The figure shows three views and two pictorial views of one solid part (mm, origin at its lowest corner). Answer the questions. Give positions to 0.01 mm unless a question says otherwise; leave off trailing zeros. Order: outer loops, then holes, each group sorted by start corner. A loop starts at its lowest first (then second) coordinate and runs counter-clockwise, first axis right, second up. Notation, with made-up numbers: M 27,50.5 L 41,50.5 A13 ccw 41,73.5 Z; hole C 62,-22 d5. An arc over 180 degrees is marked long. One line per item, written item: value.
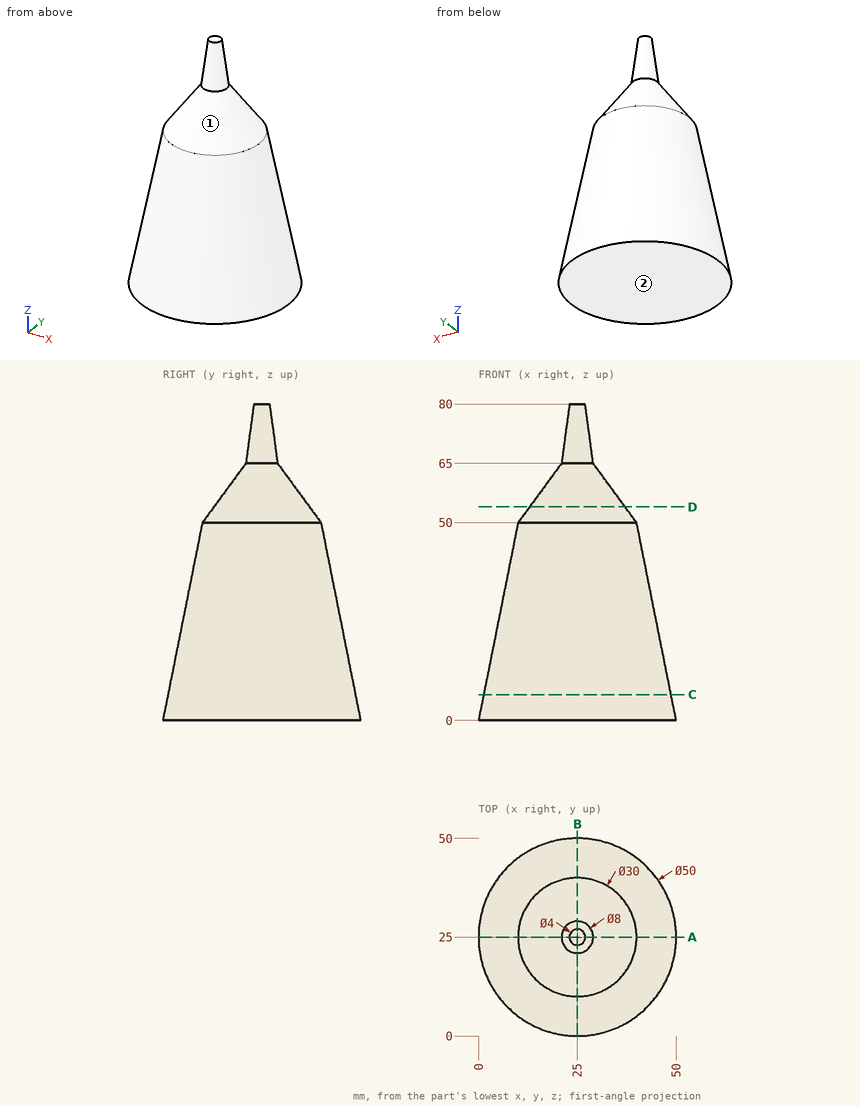
1) Determine the mould class of the marked faces 1 and 2 for opening direction Y: +Y half, -Y half, draft (parallel to the pull), parting line (faces both ways), or undercut.
Reported:
face 1: parting line
face 2: draft
2) Consider probe 1 along Y at (x, z) = (18.5, 47.5); probe 2 along Z at (x, y) = (32, 16.5); probe 3 along Y at (x, z) = (20.5, 26.5). Determine where each line is inside the solid, lowest interval first.
Reported:
probe 1: y = 10.93 to 39.07
probe 2: z = 0 to 55.44
probe 3: y = 5.82 to 44.18
3) Find section D-D, the plane z = 54. Write down the section's boundary in (x, y), plus the area to 3 significant figures.
Reported:
outline: C 25,25 d24.13
area: 457 mm^2
4) Each of these flat-tipped pins is pushed along its axis until it touches: pin 1 Ø2 at (x, y) = (26, 18) entering from +Z; pin 2 Ø12 at (x, z) = (9, 28) entering from +Y; pin 3 Ø4 at (x, z) = (36.5, 42) entering from -Y. Where does it stop, or does it pass through?
Reported:
pin 1: stops at z = 62.18
pin 2: stops at y = 41.88
pin 3: stops at y = 11.3
5) Find section C-C, the plane z = 6.5. Write down the section's boundary in (x, y).
Reported:
outline: C 25,25 d47.4
6) Find section A-A, the plane y = 25. Write down the section's boundary in (x, z).
Reported:
outline: M 0,0 L 50,0 L 40,50 L 29,65 L 27,80 L 23,80 L 21,65 L 10,50 Z
